Geometry check sheet. Reference: the model listing, model coordinates, mm. Face numbers are marked on the shaded views. A direction names the side the tool comes from. Coordinates: 2 decimals unless noted, no trailing zeros. Loops run counter-clockwise (first coordinate to the right, second up) from the corner with the lowest first, then second, coordinate; pieces in that order, holes last. Notation, with made-up numbers: (5.5, 28) - (64.5, 28) arc R33 ccw to (64.5, 61) - close; hole circle Ø4 at (24.25, 18.5). An arc over 180 degrees is marked (long way). One line per item, written item: value.
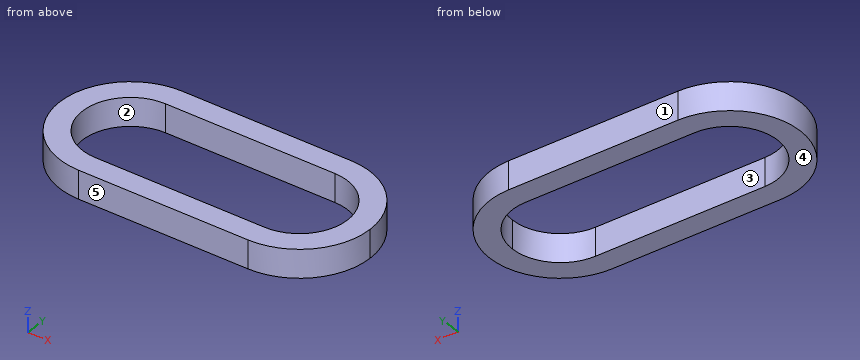
from build123d import *

# Parameters (mm, degrees)
F1_DEPTH = 5
F2_T     = -4


with BuildPart() as f1:
    # F0 (on Top) → F1 (new body)
    with BuildSketch(Plane.XY):
        with BuildLine():
            Line((-15, -12.5), (-15, 12.5))
            ThreePointArc((-15, 12.5), (-27.5, 0), (-15, -12.5))
        make_face()
        with BuildLine():
            ThreePointArc((-2.5, 0), (-6.161165, 8.838835), (-15, 12.5))
            Line((-15, 12.5), (-15, -12.5))
            ThreePointArc((-15, -12.5), (-6.161165, -8.838835), (-2.5, 0))
        make_face()
        with BuildLine():
            ThreePointArc((15, -12.5), (2.5, 0), (15, 12.5))
            Line((15, 12.5), (-15, 12.5))
            ThreePointArc((-15, 12.5), (-6.161165, 8.838835), (-2.5, 0))
            ThreePointArc((-2.5, 0), (-6.161165, -8.838835), (-15, -12.5))
            Line((-15, -12.5), (15, -12.5))
        make_face()
        with BuildLine():
            Line((15, -12.5), (15, 12.5))
            ThreePointArc((15, 12.5), (2.5, 0), (15, -12.5))
        make_face()
        with BuildLine():
            ThreePointArc((27.5, 0), (23.838835, 8.838835), (15, 12.5))
            Line((15, 12.5), (15, -12.5))
            ThreePointArc((15, -12.5), (23.838835, -8.838835), (27.5, 0))
        make_face()
    extrude(amount=F1_DEPTH)

    # F2
    f2_openings = [f1.faces().sort_by_distance(p)[0] for p in [
        (0, 0, 5),
        (0, 0, 0),
    ]]
    offset(amount=F2_T, openings=f2_openings)


solid = f1.part
(1) Cross-section at C-C on z = 2.7. Record the cut outline in (x, y).
Reply:
outline: (-15, -12.5) - (15, -12.5) arc R12.5 ccw to (27.5, 0) arc R12.5 ccw to (15, 12.5) - (-15, 12.5) arc R12.5 ccw to start; hole (-15, -8.5) - (15, -8.5) arc R8.5 ccw to (23.5, 0) arc R8.5 ccw to (15, 8.5) - (-15, 8.5) arc R8.5 ccw to start
(2) Release check for a two-part mould opening along Y. For the marked faces 3, 4 and 5 record: pulls with the +Y half, pulls with the -Y half, needs draft (parallel to the pull), parting line crosses it, or undercut.
Reply:
face 3: undercut
face 4: needs draft
face 5: pulls with the -Y half
(3) Material ranges on probe 1 along Y at (x, z) = (1.5, 4.75); probe 2 along X at (y, z) = (-3.5, 2.5); probe 3 along X at (y, z) = (7.5, 1.4), recorded low to high. Write a range as from..to.
Reply:
probe 1: -12.5..-8.5, 8.5..12.5
probe 2: -27..-22.75, 22.75..27
probe 3: -25..-19, 19..25
(4) Cross-section at A-A on x = 13. Record the cut outline in (y, z).
Reply:
outline: (-12.5, 0) - (-8.5, 0) - (-8.5, 5) - (-12.5, 5) - close; (8.5, 0) - (12.5, 0) - (12.5, 5) - (8.5, 5) - close
(5) Go/stop test with flat-tipped pins: pin 1 Ø12 at (x, y) = (-13, -9) entering from -Z; pin 2 Ø1.5 at (x, z) = (-19, 3.5) entering from -Y. Record where each tip stops, or that it passes through.
Reply:
pin 1: z = 0
pin 2: y = -12.07
(6) Access from +Z, -Z, +X, -X, +Y, -Y to the whole of each face (thin tool, end or side, straight path). Record for the marked faces 1 and 2.
Reply:
face 1: +Z, -Z, +X, -X, +Y
face 2: +Z, -Z
(7) Cross-section at B-B on y = -7.5. Record the cut outline in (x, z), and give its area (3 significant figures).
Reply:
outline: (-25, 0) - (-19, 0) - (-19, 5) - (-25, 5) - close; (19, 0) - (25, 0) - (25, 5) - (19, 5) - close
area: 60.0 mm2
